```python
from build123d import *

# Parameters (mm, degrees)
F1_DEPTH = 3


# Not quite as in the source:
# - ends of sketch curves that miss each other by under 0.0002 mm in the source are joined


with BuildPart() as f1:
    # F0 (on Front) → F1 (new body)
    with BuildSketch(Plane.XZ):
        Polygon((-86.6666681571, 50), (-100.0000014901, 50), (-100.0000014901, 53.0000007451), (-113.3729092283, 53.0000007451), (-113.3729092283, 50.0000007451), (-126.7062425613, 50.0000007451), (-126.7062425613, -50), (100, -50), (110.67250236, 50), (86.6666611759, 50), (86.6666611759, 53), (73.3333278429, 53), (73.3333278429, 50), (59.9999951759, 50), (59.9999951759, 53), (46.6666618429, 53), (46.6666618429, 50), (33.3333291759, 50), (33.3333291759, 53), (19.9999958429, 53), (19.9999958429, 50), (6.6666631759, 50), (6.6666631759, 53), (-6.6666701571, 53), (-6.6666701571, 50), (-20.0000028241, 50), (-20.0000028241, 53), (-33.3333361571, 53), (-33.3333361571, 50), (-46.6666688241, 50), (-46.6666688241, 53), (-60.0000021571, 53), (-60.0000021571, 50), (-73.3333348241, 50), (-73.3333348241, 53), (-86.6666681571, 53), align=None)
    extrude(amount=F1_DEPTH)


solid = f1.part
```
Geometry check sheet. Reference: the model listing, model coordinates, mm. Coordinates: 2 decimals unless noted, no trailing zeros. Write each loop counter-clockwise with the first axis right and the second up, starting at its lowest first coordinate (ties: lowest second). Pieces come first, ordered by that corner, then holes. Notation, with made-up numbers: (45, -12) -> (99, -12) arc R25 cw to (99, 6) -> close; hole circle Ø10 at (63, 12). An arc over 180 degrees is marked (long way). Use CSV: the item, a comma, the result in double quotes. Start each with the question number.
Item 1: Cross-section at B-B, the plane z = -10.5. Record the cut outline in (x, y).
Item 2: Cross-section at A-A, the plane x = 39. Record the cut outline in (y, z), plus the area to 3 significant figures.
Item 3: Thickness scan on line 1 (Z direction, x = 62, y = -2.65); line 2 (X direction, y = -0.7, z = 28); line 3 (X direction, y = -0.65, z = -32). Record the ranges inside material, lowest first.
Item 4: Depth check by flat-ended pin: pin 1 Ø1.5 at (y, z) = (-1.5, 51) entering from +X; pin 2 Ø1.5 at (x, y) = (12, -1.5) entering from +Z; pin 3 Ø12 at (x, z) = (52.5, -4.5) entering from +Y; pin 4 Ø1.5 at (y, z) = (-2, 51) entering from -X. Enter the tip coordinate at first touch or a pass-through.
Answers:
1,outline,"(-126.71, -3) -> (104.22, -3) -> (104.22, 0) -> (-126.71, 0) -> close"
2,outline,"(-3, -50) -> (0, -50) -> (0, 50) -> (-3, 50) -> close"
2,area,"300 mm^2"
3,line 1,"-50 to 50"
3,line 2,"-126.71 to 108.32"
3,line 3,"-126.71 to 101.92"
4,pin 1,"x = 86.67"
4,pin 2,"z = 50"
4,pin 3,"y = 0"
4,pin 4,"x = -113.37"
